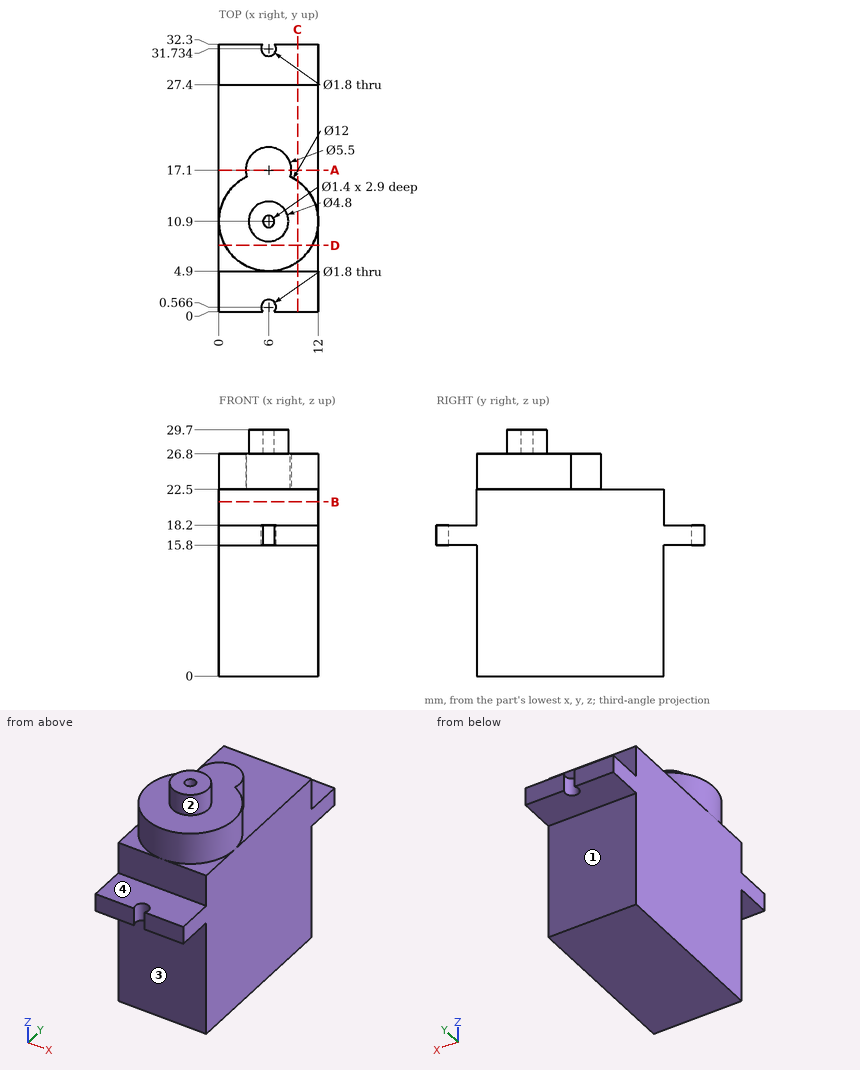
Study the drawing (mm; zero at the part's minimum x, y, z) and answer. A direction names the side the tool comes from. Round coordinates to 2 decimals unless told otherwise and drop trailing zeros. Write each loop counter-clockwise with the first axis right and the second up, starting at its lowest first coordinate (ties: lowest second). Pieces come first, ordered by that corner, then holes. Notation, with made-up numbers: (4.25, 73.5) -> (51.25, 73.5) arc R20 ccw to (51.25, 100.5) -> close; hole circle Ø3 at (-9, 53). An arc over 180 degrees is marked (long way). Write item = value, one per line.
1) Section B-B on z = 21 is taken. Write down the section's boundary in (x, y), plus the area to 3 significant figures.
Check values:
outline = (0, 4.9) -> (12, 4.9) -> (12, 27.4) -> (0, 27.4) -> close
area = 270 mm²
2) Given pin 1 (1.5 mm diameter, centred on x = 4.5, y = 1.5, fed in from +Z); pin 2 (6 mm diameter, centred on x = 2.5, y = 17.5, fed in from +Z); pin 3 (1.1 mm diameter, centred on x = 6, y = 31.73, fed in from +Z); pin 4 (1.3 mm diameter, centred on x = 5.5, z = 19.5, fed in from -Y), each flat-ended and moving along its own axis, determine where each tip first touches the part or whether it passes through.
Check values:
pin_1 = 18.2
pin_2 = 26.8
pin_3 = through
pin_4 = 4.9
3) Which of the six approach directions +Z, -Z, +X, -X, +Y, -Y give full straight-line access (tool end or side, diameter ignored) to the marked faces 1, 2, 3 and 4?
Check values:
face_1 = -Z, +X, -X, +Y
face_2 = +Z
face_3 = -Z, +X, -X, -Y
face_4 = +Z, +X, -X, -Y
4) Straight lines are drawn through the part: line 1 along Z through (x, y) = (9.25, 31); line 2 along Z through (x, y) = (5, 17); line 3 along Y through (x, z) = (9.5, 7.5). For each, find the intervals that lie inside material, in ascending order. Write a range as [from, to].
Check values:
line_1 = [15.8, 18.2]
line_2 = [0, 26.8]
line_3 = [4.9, 27.4]
5) Section C-C on x = 9.5 is taken. Write down the section's boundary in (y, z), plus the area to 3 significant figures.
Check values:
outline = (0, 15.8) -> (4.9, 15.8) -> (4.9, 0) -> (27.4, 0) -> (27.4, 15.8) -> (32.3, 15.8) -> (32.3, 18.2) -> (27.4, 18.2) -> (27.4, 22.5) -> (15.77, 22.5) -> (15.77, 26.8) -> (6.03, 26.8) -> (6.03, 22.5) -> (4.9, 22.5) -> (4.9, 18.2) -> (0, 18.2) -> close
area = 572 mm²
6) Section A-A on y = 17.1 is taken. Write down the section's boundary in (x, z), plus the area to 3 significant figures.
Check values:
outline = (0, 0) -> (12, 0) -> (12, 22.5) -> (8.75, 22.5) -> (8.75, 26.8) -> (3.25, 26.8) -> (3.25, 22.5) -> (0, 22.5) -> close
area = 294 mm²
7) Section D-D on y = 8 is taken. Write down the section's boundary in (x, z).
Check values:
outline = (0, 0) -> (12, 0) -> (12, 22.5) -> (11.25, 22.5) -> (11.25, 26.8) -> (0.75, 26.8) -> (0.75, 22.5) -> (0, 22.5) -> close
